from build123d import *

# Parameters (mm, degrees)
SKETCH1_W                                       = 420
SKETCH1_H                                       = 250
BOSS_EXTRUDE1_DEPTH                             = 10
CHAMFER1_SIZE                                   = 2.5
CSK_FOR_M3_FLAT_HEAD_MACHINE_SCREW2_D           = 3.4
CSK_FOR_M3_FLAT_HEAD_MACHINE_SCREW2_DEPTH       = 15
CSK_FOR_M3_FLAT_HEAD_MACHINE_SCREW2_CSINK_D     = 6.3
CSK_FOR_M3_FLAT_HEAD_MACHINE_SCREW2_CSINK_ANGLE = 90
CSK_FOR_M3_FLAT_HEAD_MACHINE_SCREW2_TIP         = 1.021463052
SKETCH7_OUTSIDE_W                               = 519.776
SKETCH7_OUTSIDE_H                               = 349.776
SKETCH7_OUTSIDE_W_2                             = 400
SKETCH7_OUTSIDE_H_2                             = 230
CUT_EXTRUDE2_DEPTH                              = 5
CHAMFER2_SIZE                                   = 2.5
F_10_0MM_DOWEL_HOLE1_D                          = 10
F_1_0MM_DOWEL_HOLE1_D                           = 1


with BuildPart() as part:
    # Sketch1 → Boss-Extrude1 (new body)
    with BuildSketch(Plane.XY):
        with Locations((190, 105)):
            Rectangle(SKETCH1_W, SKETCH1_H)
    extrude(amount=-BOSS_EXTRUDE1_DEPTH)

    # Chamfer1
    chamfer1_edges = [part.edges().sort_by_distance(p)[0] for p in [
        (-20, 230, -5),
        (400, 230, -5),
        (400, -20, -5),
        (-20, -20, -5),
    ]]
    chamfer(chamfer1_edges, length=CHAMFER1_SIZE)

    # CSK for M3 Flat Head Machine Screw2
    with Locations(Plane.XY):
        with Locations((-15, 225), (190, 225), (395, 225), (395, -15), (190, -15), (-15, -15), (-15, 105), (395, 105)):
            CounterSinkHole(CSK_FOR_M3_FLAT_HEAD_MACHINE_SCREW2_D / 2, CSK_FOR_M3_FLAT_HEAD_MACHINE_SCREW2_CSINK_D / 2, depth=CSK_FOR_M3_FLAT_HEAD_MACHINE_SCREW2_DEPTH, counter_sink_angle=CSK_FOR_M3_FLAT_HEAD_MACHINE_SCREW2_CSINK_ANGLE)
            with Locations((0, 0, -(CSK_FOR_M3_FLAT_HEAD_MACHINE_SCREW2_DEPTH + CSK_FOR_M3_FLAT_HEAD_MACHINE_SCREW2_TIP / 2))):  # 118° drill point
                Cone(0, CSK_FOR_M3_FLAT_HEAD_MACHINE_SCREW2_D / 2, CSK_FOR_M3_FLAT_HEAD_MACHINE_SCREW2_TIP, mode=Mode.SUBTRACT)

    # Sketch7 outside → Cut-Extrude2 (cut)
    with BuildSketch(Plane(origin=(0, 0, -10), x_dir=(-1, 0, 0), z_dir=(0, 0, -1))):
        with Locations((-190, 105)):
            Rectangle(SKETCH7_OUTSIDE_W, SKETCH7_OUTSIDE_H)
        with Locations((-190, 105)):
            Rectangle(SKETCH7_OUTSIDE_W_2, SKETCH7_OUTSIDE_H_2, mode=Mode.SUBTRACT)
    extrude(amount=-CUT_EXTRUDE2_DEPTH, mode=Mode.SUBTRACT)

    # Chamfer2
    chamfer2_edges = [part.edges().sort_by_distance(p)[0] for p in [
        (-10, -10, -7.5),
        (390, -10, -7.5),
        (390, 220, -7.5),
        (-10, 220, -7.5),
    ]]
    chamfer(chamfer2_edges, length=CHAMFER2_SIZE)

    # Ø10.0mm Dowel Hole1 (through all)
    with Locations(Plane.XY):
        with Locations((0, 210)):
            f_10_0mm_dowel_hole1 = Hole(F_10_0MM_DOWEL_HOLE1_D / 2)

    # Mirror1: Ø10.0mm Dowel Hole1 across plane
    add(f_10_0mm_dowel_hole1.mirror(Plane.ZY.offset(-190)), mode=Mode.SUBTRACT)

    # Ø1.0mm Dowel Hole1 (through all)
    with Locations(Plane.XY):
        with Locations((-15, 165), (395, 45)):
            Hole(F_1_0MM_DOWEL_HOLE1_D / 2)


solid = part.part
Model file for the job. Use its own axes, mm. A direction names the side the tool comes from. Give positions to 0.01 mm unless a question says otherwise; leave off trailing zeros. Loops run counter-clockwise (first coordinate to the right, second up) from the corner with the lowest first, then second, coordinate; pieces in that order, holes last.
1) Saw through at C-C (x = 28.5). Write the cut outline in (y, z).
2) Tool access for faces 3 (the flat face through (207, -15, -5)), 4 (the cylindrical face through (0.651, 214.957, -5.07)): list every direction of +Z, -Z, +X, -X, +Y, -Y with a clear straight run to the whole face (end or side of a thin tool).
3) Flat gauge pins, fed straight in: pin 1 Ø5.5 at (y, z) = (60, -6.5) entering from -X; pin 2 Ø2.5 at (x, y) = (395, 105) entering from +Z; pin 3 Ø2.5 at (y, z) = (138, -7.5) entering from +X; pin 4 Ø1.5 at (x, z) = (108.5, -8) entering from +Y. Where does each tip first touch, or does it go through?
4) Saw through at B-B (y = 128.5). Write the cut outline in (x, z), plus the area to 3 significant figures.
5) Pull direction Y, two halves, no side cores. Call faces 1 (the cylindrical face through (384.77, 211.5, -5.07)), 2 (the flat face through (187, 107, -10)): +Y half, -Y half, draft (parallel to the pull), parting line (faces both ways), or undercut.
6) Saw through at A-A (z = -7.75). Write the cut outline in (x, y).
7) Wall check: line 1 (Y direction, x = -15, z = -4.25); line 2 (X direction, y = -15, z = -3.1); line 3 (X direction, y = 105, z = -2.65). Give the ranges that are in metal, low to high.
Answer block:
1. outline: (-20, -5) - (-10, -5) - (-10, -10) - (220, -10) - (220, -5) - (230, -5) - (230, 0) - (-20, 0) - close
2. face 3: -Z
2. face 4: +Z, -Z
3. pin 1: stops at x = -20
3. pin 2: passes through
3. pin 3: stops at x = 390
3. pin 4: stops at y = 220
4. outline: (-20, -5) - (-10, -5) - (-10, -10) - (390, -10) - (390, -5) - (400, -5) - (400, 0) - (-20, 0) - close
4. area: 4,100 mm2
5. face 1: undercut
5. face 2: draft
6. outline: (-10, -7.5) - (-7.5, -10) - (387.5, -10) - (390, -7.5) - (390, 217.5) - (387.5, 220) - (-7.5, 220) - (-10, 217.5) - close; hole circle Ø10 at (0, 210); hole circle Ø10 at (380, 210)
7. line 1: y = -20 to -16.7, -13.3 to 103.3, 106.7 to 164.5, 165.5 to 223.3, 226.7 to 230
7. line 2: x = -20 to -16.7, -13.3 to 188.3, 191.7 to 393.3, 396.7 to 400
7. line 3: x = -20 to -16.7, -13.3 to 393.3, 396.7 to 400
